Here's how the part is built. I have some questions about the finished solid (model axes, mm). Round coordinates to 2 decimals unless told otherwise and drop trailing zeros. Loops run counter-clockwise (first coordinate to the right, second up) from the corner with the lowest first, then second, coordinate; pieces in that order, holes last. Notation, with made-up numbers: (15.5, -24.75) - (45.5, -24.75) arc R22 cw to (45.5, -8.75) - close; hole circle Ø8 at (37.25, 88). An arc over 180 degrees is marked (long way). Answer as a JSON object with one key per item and string values. Group by question number.
1) Will this pin go through, and if not, where does the flat tip stop? P1, Ø1, axis at y = 1.5, z = 10, coming from the +X side.
2) If I drill on line 1 along Z through (x, y) = (-12.5, 2.5) (3 decimals); line 2 along X through (y, z) = (2.45, -11), over which ranges is the centre line in solid material (lowest first)? Write a range as [from, to].
3) I want a section at A-A, the plane x = 22.5. Please give me the cut outline in (y, z) (3 decimals), then the cut area to 3 significant figures.
4) I want a section at B-B, the plane z = 0. Please give me the cut outline in (x, y) (3 decimals), then the cut area to 3 significant figures.
from build123d import *

# Parameters (mm, degrees)
SKETCH1_W           = 80
SKETCH1_H           = 80
BOSS_EXTRUDE1_DEPTH = 3.175
SKETCH3_OUTSIDE_W   = 104.636
SKETCH3_OUTSIDE_H   = 104.636
CUT_EXTRUDE1_DEPTH  = 57.657573413
SKETCH8_W           = 80
SKETCH8_H           = 5.333333333
BOSS_EXTRUDE2_DEPTH = 3.175


with BuildPart() as part:
    # Sketch1 → Boss-Extrude1 (new body)
    with BuildSketch(Plane(origin=(0, 0, 0), x_dir=(1, 0, 0), z_dir=(0, 1, 0))):
        Rectangle(SKETCH1_W, SKETCH1_H)
    extrude(amount=BOSS_EXTRUDE1_DEPTH)

    # Sketch3 outside → Cut-Extrude1 (cut, through all)
    with BuildSketch(Plane(origin=(0, 3.175, 0), x_dir=(1, 0, 0), z_dir=(0, 1, 0))):
        Rectangle(SKETCH3_OUTSIDE_W, SKETCH3_OUTSIDE_H)
        Polygon((-40, -40), (-34.666666667, -40), (-34.666666667, -36.825), (-29.333333333, -36.825), (-29.333333333, -40), (-24, -40), (-24, -36.825), (-18.666666667, -36.825), (-18.666666667, -40), (-13.333333333, -40), (-13.333333333, -36.825), (-8, -36.825), (-8, -40), (-2.666666667, -40), (-2.666666667, -36.825), (2.666666667, -36.825), (2.666666667, -40), (8, -40), (8, -36.825), (13.333333333, -36.825), (13.333333333, -40), (18.666666667, -40), (18.666666667, -36.825), (24, -36.825), (24, -40), (29.333333333, -40), (29.333333333, -36.825), (34.666666667, -36.825), (34.666666667, -40), (40, -40), (40, -34.666666667), (36.613333333, -34.666666667), (36.613333333, -29.333333333), (40, -29.333333333), (40, -24), (36.613333333, -24), (36.613333333, -18.666666667), (40, -18.666666667), (40, -13.333333333), (36.613333333, -13.333333333), (36.613333333, -8), (40, -8), (40, -2.666666667), (36.613333333, -2.666666667), (36.613333333, 2.666666667), (40, 2.666666667), (40, 8), (36.613333333, 8), (36.613333333, 13.333333333), (40, 13.333333333), (40, 18.666666667), (36.613333333, 18.666666667), (36.613333333, 24), (40, 24), (40, 29.333333333), (36.613333333, 29.333333333), (36.613333333, 34.666666667), (40, 34.666666667), (40, 40), (34.666666667, 40), (34.666666667, 36.825), (29.333333333, 36.825), (29.333333333, 40), (24, 40), (24, 36.825), (18.666666667, 36.825), (18.666666667, 40), (13.333333333, 40), (13.333333333, 36.825), (8, 36.825), (8, 40), (2.666666667, 40), (2.666666667, 36.825), (-2.666666667, 36.825), (-2.666666667, 40), (-8, 40), (-8, 36.825), (-13.333333333, 36.825), (-13.333333333, 40), (-18.666666667, 40), (-18.666666667, 36.825), (-24, 36.825), (-24, 40), (-29.333333333, 40), (-29.333333333, 36.825), (-34.666666667, 36.825), (-34.666666667, 40), (-40, 40), (-40, 34.666666667), (-36.613333333, 34.666666667), (-36.613333333, 29.333333333), (-40, 29.333333333), (-40, 24), (-36.613333333, 24), (-36.613333333, 18.666666667), (-40, 18.666666667), (-40, 13.333333333), (-36.613333333, 13.333333333), (-36.613333333, 8), (-40, 8), (-40, 2.666666667), (-36.613333333, 2.666666667), (-36.613333333, -2.666666667), (-40, -2.666666667), (-40, -8), (-36.613333333, -8), (-36.613333333, -13.333333333), (-40, -13.333333333), (-40, -18.666666667), (-36.613333333, -18.666666667), (-36.613333333, -24), (-40, -24), (-40, -29.333333333), (-36.613333333, -29.333333333), (-36.613333333, -34.666666667), (-40, -34.666666667), align=None, mode=Mode.SUBTRACT)
    extrude(amount=-CUT_EXTRUDE1_DEPTH, mode=Mode.SUBTRACT)

    # Sketch8 → Boss-Extrude2 (add)
    with BuildSketch(Plane(origin=(0, 3.175, 0), x_dir=(1, 0, 0), z_dir=(0, 1, 0))):
        with Locations((0, 37.333333334)):
            Rectangle(SKETCH8_W, SKETCH8_H)
    extrude(amount=-BOSS_EXTRUDE2_DEPTH)


solid = part.part
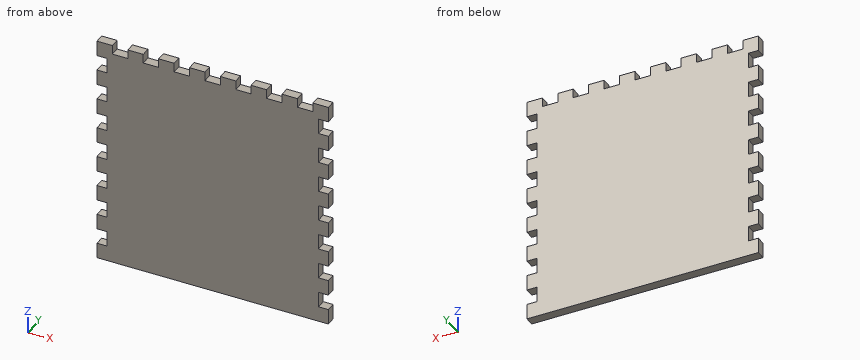
Outcome:
{
 "1": {"P1": "x = 36.61"},
 "2": {"line 1": "[-40, 36.825]", "line 2": "[-36.61, 36.61]"},
 "3": {"outline": "(0, -40) - (3.175, -40) - (3.175, 36.825) - (0, 36.825) - close", "area": "244 mm^2"},
 "4": {"outline": "(-36.613, 0) - (36.613, 0) - (36.613, 3.175) - (-36.613, 3.175) - close", "area": "232 mm^2"}
}
